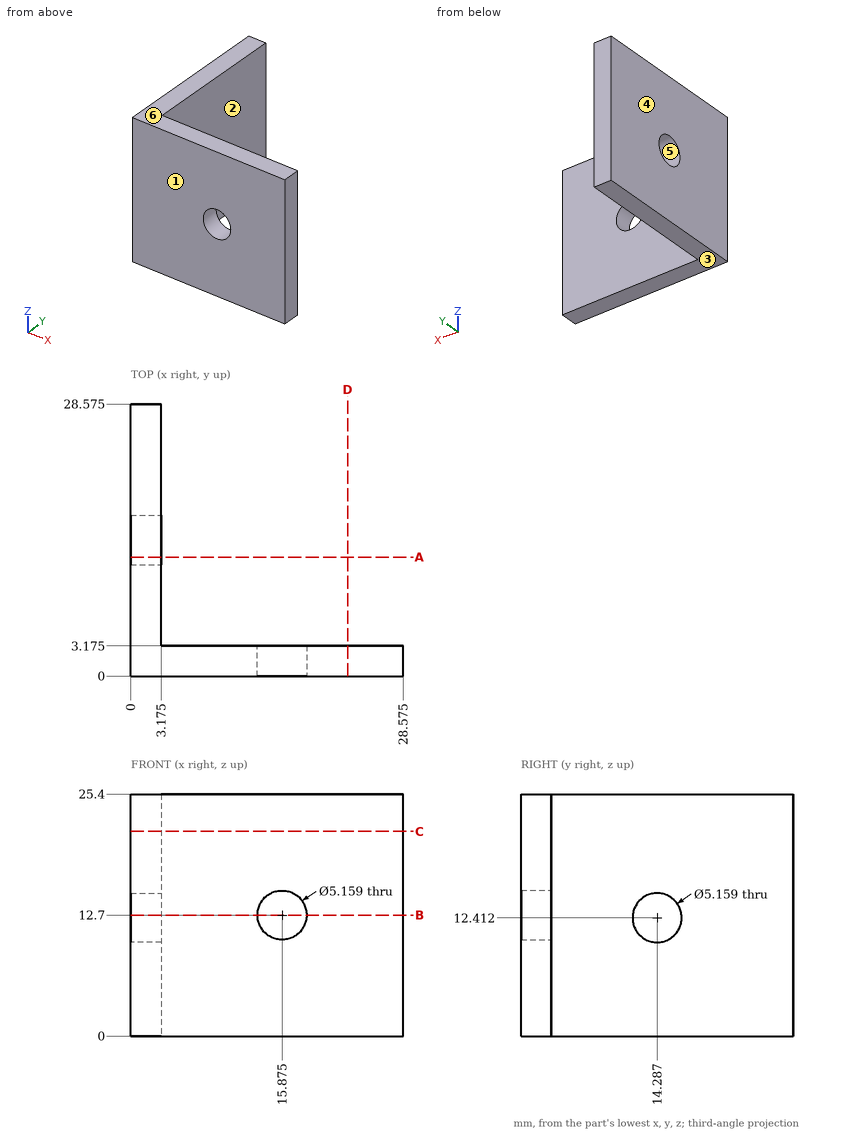
Verification items for this drawing (mm, ordinates from the low corner). A direction names the side the tool comes from. Coordinates: 2 decimals unless noted, no trailing zeros. Write each loop counter-clockwise with the first axis right and the second up, starting at its lowest first coordinate (ties: lowest second). Pieces come first, ordered by that corner, then holes. Notation, with made-up numbers: M -16.5,60 L -6.5,60 A31 cw -6.5,88 Z; hole C 9,3.5 d7. An arc over 180 degrees is marked long. One line per item, written item: value. Start each with the question number.
(1) Sectioned sample at B-B, the plane z = 12.7. Enter the section's corners in (x, y) (1 decimal).
(2) Release check for a two-part mould opening along Z. For the marked faces 3, 4, 5 and 6 record: released by +Z, released by -Z, zero draft, split by the parting line, or undercut.
(3) Sectioned sample at D-D, the plane x = 22.75. Enter the section's corners in (y, z) (1 decimal).
(4) Tool access check on the marked faces 1 and 2. Record the directions out of +Z, -Z, +X, -X, +Y, -Y that give a thin tool (end or side, any length) a straight path to the whole face; none if there is none.
(5) Scan lines: line 1 along X through (y, z) = (2.05, 12.7) (1 decimal); line 2 along X through (y, z) = (7, 17.5) (1 decimal). Record each from-to range of solid material in increasing order. Write a range as [from, to].
(6) Sectioned sample at C-C, the plane z = 21.5. Enter the section's corners in (x, y) (1 decimal).
(7) Sectioned sample at A-A, the plane y = 12.5. Enter the section's corners in (x, z) (1 decimal).
(8) Depth check by flat-ended pin: pin 1 (2 mm diameter, centred on x = 17.5, z = 13.5, fed in from -Y); pin 2 (1 mm diameter, centred on y = 20, z = 21, fed in from +X) (1 decimal); pin 3 (7.5 mm diameter, centred on x = 18.5, z = 11.5, fed in from +Y) (1 decimal). Enter the tip coordinate at first touch or a pass-through.
Filled sheet:
1. outline: M 0,0 L 13.3,0 L 13.3,3.2 L 3.2,3.2 L 3.2,11.7 L 0,11.7 Z; M 0,16.9 L 3.2,16.9 L 3.2,28.6 L 0,28.6 Z; M 18.5,0 L 28.6,0 L 28.6,3.2 L 18.5,3.2 Z
2. face 3: released by -Z
2. face 4: zero draft
2. face 5: undercut
2. face 6: released by +Z
3. outline: M 0,0 L 3.2,0 L 3.2,25.4 L 0,25.4 Z
4. face 1: +Z, -Z, +X, -X, -Y
4. face 2: +Z, -Z, +X, +Y
5. line 1: [0, 13.3], [18.5, 28.6]
5. line 2: [0, 3.2]
6. outline: M 0,0 L 28.6,0 L 28.6,3.2 L 3.2,3.2 L 3.2,28.6 L 0,28.6 Z
7. outline: M 0,0 L 3.2,0 L 3.2,10.6 L 0,10.6 Z; M 0,14.3 L 3.2,14.3 L 3.2,25.4 L 0,25.4 Z
8. pin 1: y = 0
8. pin 2: x = 3.2
8. pin 3: y = 3.2
